```python
from build123d import *

# Parameters (mm, degrees)
F0_R     = 4.25
F0_R_2   = 2.25
F1_DEPTH = 4
F2_DEPTH = 1.5
F3_R     = 4.75
F3_R_2   = 2.25
F4_DEPTH = 2


with BuildPart() as f1:
    # F0 (on Top) → F1 (new body)
    with BuildSketch(Plane.XY):
        with BuildLine():
            ThreePointArc((-65, -60), (-63.5355339059, -63.5355339059), (-60, -65))
            Line((-60, -65), (60, -65))
            ThreePointArc((60, -65), (63.5355339059, -63.5355339059), (65, -60))
            Line((65, -60), (65, 60))
            ThreePointArc((65, 60), (63.5355339059, 63.5355339059), (60, 65))
            Line((60, 65), (-60, 65))
            ThreePointArc((-60, 65), (-63.5355339059, 63.5355339059), (-65, 60))
            Line((-65, 60), (-65, -60))
        make_face()
        with Locations((-50, -50)):
            Circle(F0_R, mode=Mode.SUBTRACT)
        with Locations((50, -50)):
            Circle(F0_R, mode=Mode.SUBTRACT)
        with Locations((-50, 50)):
            Circle(F0_R, mode=Mode.SUBTRACT)
        with Locations((50, 50)):
            Circle(F0_R, mode=Mode.SUBTRACT)
        with Locations((-50, -50)):
            Circle(F0_R)
        with Locations((-50, -50)):
            Circle(F0_R_2, mode=Mode.SUBTRACT)
        with Locations((50, -50)):
            Circle(F0_R)
        with Locations((50, -50)):
            Circle(F0_R_2, mode=Mode.SUBTRACT)
        with Locations((50, 50)):
            Circle(F0_R)
        with Locations((50, 50)):
            Circle(F0_R_2, mode=Mode.SUBTRACT)
        with Locations((-50, 50)):
            Circle(F0_R)
        with Locations((-50, 50)):
            Circle(F0_R_2, mode=Mode.SUBTRACT)
    extrude(amount=F1_DEPTH)

    # F0 (on Top) → F2 (join)
    with BuildSketch(Plane.XY):
        with Locations((50, -50)):
            Circle(F0_R)
        with Locations((50, -50)):
            Circle(F0_R_2, mode=Mode.SUBTRACT)
        with Locations((50, 50)):
            Circle(F0_R)
        with Locations((50, 50)):
            Circle(F0_R_2, mode=Mode.SUBTRACT)
        with Locations((-50, 50)):
            Circle(F0_R)
        with Locations((-50, 50)):
            Circle(F0_R_2, mode=Mode.SUBTRACT)
        with Locations((-50, -50)):
            Circle(F0_R)
        with Locations((-50, -50)):
            Circle(F0_R_2, mode=Mode.SUBTRACT)
    extrude(amount=-F2_DEPTH)

    # F3 (on face) → F4 (cut)
    with BuildSketch(Plane.XY.offset(4)):
        with Locations((-50, 50)):
            Circle(F3_R)
        with Locations((-50, 50)):
            Circle(F3_R_2, mode=Mode.SUBTRACT)
        with Locations((50, 50)):
            Circle(F3_R)
        with Locations((50, 50)):
            Circle(F3_R_2, mode=Mode.SUBTRACT)
        with Locations((50, -50)):
            Circle(F3_R)
        with Locations((50, -50)):
            Circle(F3_R_2, mode=Mode.SUBTRACT)
        with Locations((-50, -50)):
            Circle(F3_R)
        with Locations((-50, -50)):
            Circle(F3_R_2, mode=Mode.SUBTRACT)
    extrude(amount=-F4_DEPTH, mode=Mode.SUBTRACT)


solid = f1.part
```
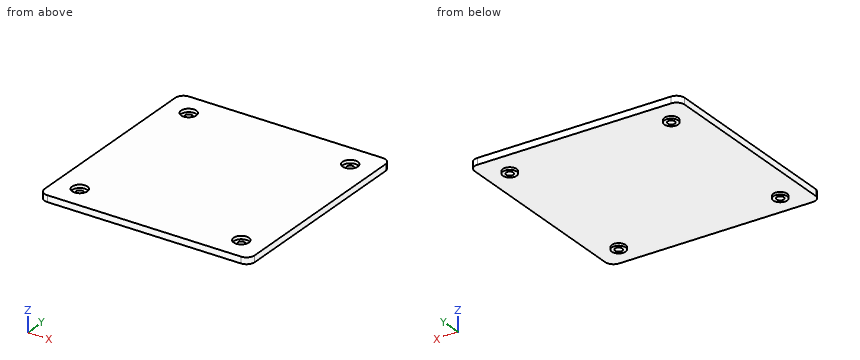
Input: part model. Units: mm. Frame: model coordinates. Coordinates: 2 decimals unless noted, no trailing zeros. Loops run counter-clockwise (first coordinate to the right, second up) from the corner with the lowest first, then second, coordinate; pieces in that order, holes last. Notation, with made-up numbers: M 21.25,-32 L 30.25,-32 A15 cw 30.25,-24 Z; hole C -2,34.25 d8. An arc over 180 degrees is marked long. Answer in a Markdown table with one row per item.
1. Section D-D, the plane x = -17. Output: boundary loops of the cut face in (y, z), then the cut area to 3 significant figures.
Response:
| item | result |
|---|---|
| outline | M -65,0 L 65,0 L 65,4 L -65,4 Z |
| area | 520 mm2 |
2. Section A-A, the plane x = -50. Output: boundary loops of the cut face in (y, z).
Response:
| item | result |
|---|---|
| outline | M -65,0 L -54.25,0 L -54.25,-1.5 L -52.25,-1.5 L -52.25,2 L -54.75,2 L -54.75,4 L -65,4 Z; M -47.75,-1.5 L -45.75,-1.5 L -45.75,0 L 45.75,0 L 45.75,-1.5 L 47.75,-1.5 L 47.75,2 L 45.25,2 L 45.25,4 L -45.25,4 L -45.25,2 L -47.75,2 Z; M 52.25,-1.5 L 54.25,-1.5 L 54.25,0 L 65,0 L 65,4 L 54.75,4 L 54.75,2 L 52.25,2 Z |
3. First-contact query: pin 1 (3 mm diameter, centred on x = -49, y = -50, fed in from +Z); pin 2 (4 mm diameter, centred on x = -27.5, y = 38, fed in from -Z). Flat tips, straight axial feed; report the tip coordinate or a pass-through.
Response:
| item | result |
|---|---|
| pin 1 | stops at z = 2 |
| pin 2 | stops at z = 0 |
4. Section B-B, the plane z = 3. Output: boundary loops of the cut face in (x, y).
Response:
| item | result |
|---|---|
| outline | M -65,-60 A5 ccw -60,-65 L 60,-65 A5 ccw 65,-60 L 65,60 A5 ccw 60,65 L -60,65 A5 ccw -65,60 Z; hole C -50,-50 d9.5; hole C -50,50 d9.5; hole C 50,-50 d9.5; hole C 50,50 d9.5 |
5. Material intervals for line 1 (Y direction, x = 50, z = -0.5); line 2 (Y direction, x = 50, z = 2.5); line 3 (Z direction, x = -29.5, y = -14), sorted ascending.
Response:
| item | result |
|---|---|
| line 1 | y = -54.25 to -52.25, -47.75 to -45.75, 45.75 to 47.75, 52.25 to 54.25 |
| line 2 | y = -65 to -54.75, -45.25 to 45.25, 54.75 to 65 |
| line 3 | z = 0 to 4 |
